Could you check a few things on this drawing? It's one solid part, dimensions in mm from its lowest x, y, z. Coordinates: 2 decimals unless noted, no trailing zeros. Loops run counter-clockwise (first coordinate to the right, second up) from the corner with the lowest first, then second, coordinate; pieces in that order, holes last. Notation, with made-up numbers: M 38.25,87 L 64.25,87 A37 cw 64.25,125 Z; hole C -4.75,70 d1. An arc over 180 degrees is marked long. Use one line per item in the form item = value. Start each with the question number.
(1) Imagine slicing it at B-B, the plane x = 33.5. Please give me the cut outline in (y, z).
(2) Please list where these lines run through material, in increasing order: L1, parallel to Y at x = 6, z = 0.9; L2, parallel to Y at x = 19.5, z = 1.2; L3, parallel to Y at x = 33.5, z = 1.5.
(3) Imagine slicing it at D-D, the plane x = 4.5. Please give me the cut outline in (y, z).
(4) Imagine slicing it at C-C, the plane y = 7. Please give me the cut outline in (x, z), and give its area (3 significant figures).
(5) Thinking about a two-plate mould opening in Y: for the marked faces 1, 2, 3 and 4, which applies, +Y half, -Y half, draft (parallel to the pull), parting line (faces both ways), or undercut?
(6) Imagine slicing it at A-A, the plane z = 3.1. State how many separate pieces and enclosed holes the cut face has, and give its area (3 significant figures).
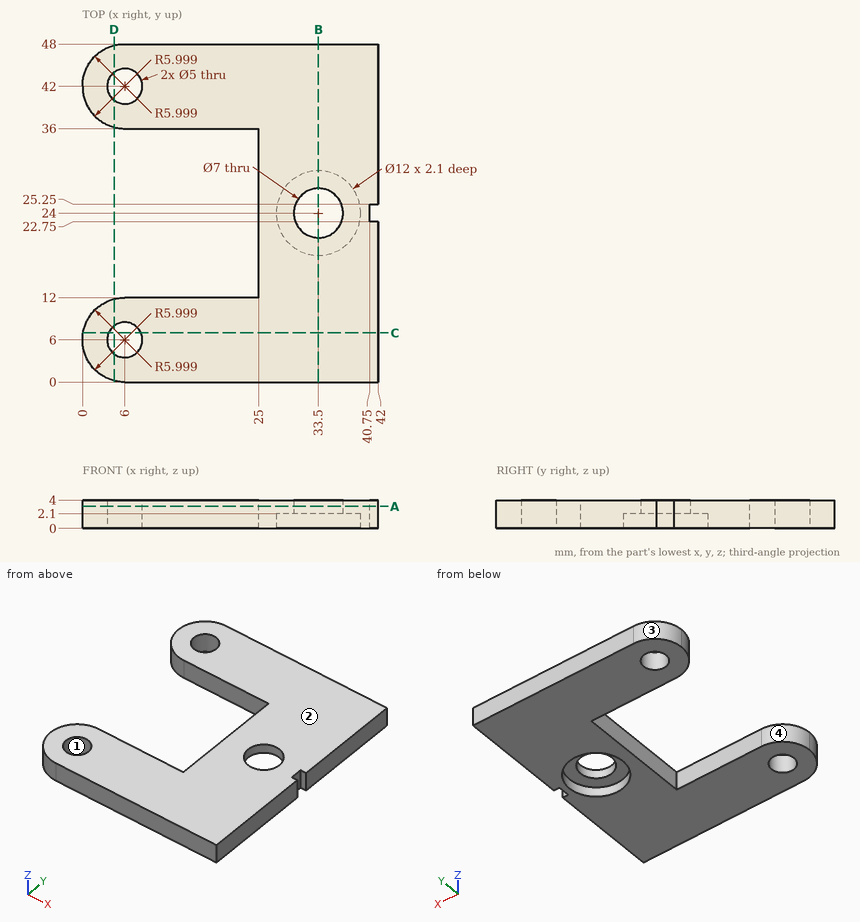
Answer:
q1.outline = M 0,0 L 18,0 L 18,2.1 L 20.5,2.1 L 20.5,4 L 0,4 Z; M 27.5,2.1 L 30,2.1 L 30,0 L 48,0 L 48,4 L 27.5,4 Z
q2.L1 = 0 to 3.5, 8.5 to 12, 36 to 39.5, 44.5 to 48
q2.L2 = 0 to 12, 36 to 48
q2.L3 = 0 to 18, 30 to 48
q3.outline = M 0.19,0 L 4,0 L 4,4 L 0.19,4 Z; M 8,0 L 11.81,0 L 11.81,4 L 8,4 Z; M 36.19,0 L 40,0 L 40,4 L 36.19,4 Z; M 44,0 L 47.81,0 L 47.81,4 L 44,4 Z
q4.outline = M 0.08,0 L 3.71,0 L 3.71,4 L 0.08,4 Z; M 8.29,0 L 42,0 L 42,4 L 8.29,4 Z
q4.area = 149 mm²
q5.face_1 = undercut
q5.face_2 = draft
q5.face_3 = +Y half
q5.face_4 = undercut
q6.separate_pieces = 1
q6.enclosed_holes = 3
q6.area = 1,300 mm²
